```python
from build123d import *

# Parameters (mm, degrees)
F1_DEPTH = 25


with BuildPart() as f1:
    # F0 (on Front) → F1 (new body)
    with BuildSketch(Plane.XZ):
        with BuildLine():
            Line((-24.272264, 6.957319), (-24.272264, -8.5))
            Line((-24.272264, -8.5), (-4.272264, -8.5))
            Line((-4.272264, -8.5), (-4.272264, -5))
            Line((-4.272264, -5), (10.727736, -5))
            Line((10.727736, -5), (10.727736, -11))
            Line((10.727736, -11), (15.727736, -11))
            Line((15.727736, -11), (15.727736, -19.5))
            Line((15.727736, -19.5), (25.727736, -19.5))
            Line((25.727736, -19.5), (25.727736, 19))
            Line((25.727736, 19), (15.727736, 19))
            Line((15.727736, 19), (15.727736, 10))
            Line((15.727736, 10), (10.727736, 10))
            ThreePointArc((10.727736, 10), (9.263269, 6.464466), (5.727736, 5))
            Line((5.727736, 5), (-4.272264, 5))
            Line((-4.272264, 5), (-4.272264, 8.5))
            Line((-4.272264, 8.5), (-20.272264, 8.5))
            Line((-20.272264, 8.5), (-24.272264, 6.957319))
        make_face()
    extrude(amount=F1_DEPTH)


solid = f1.part
```
Work out the finished part from the listing and answer in its coordinate system (mm). A direction names the side the tool comes from. Coordinates: 2 decimals unless noted, no trailing zeros. Write each loop counter-clockwise with the first axis right and the second up, starting at its lowest first coordinate (ties: lowest second). Pieces come first, ordered by that corner, then holes.
Q1. Find the intervals of material crossed by line 1 (X direction, y = -11.75, z = -7); line 2 (X direction, y = -20.25, z = -16); line 3 (Z direction, x = 0, y = -5.5), in increasing order.
Q2. A cutting plane is placed at B-B, the plane z = -9.5. Give the vertices of the cut face in (x, y).
Q3. Which of the six approach directions +Z, -Z, +X, -X, +Y, -Y give full straight-line access (tool end or side, diameter ignored) to faces 1 (the face through (3, -12, -5)), 2 (the face through (15.728, -12, -15)), 3 (the face through (9.3, -12.3, 6.5))?
Q4. Each of these flat-tipped pins is pushed along its axis until it touches: pin 1 Ø6 at (y, z) = (-3, -10) entering from -X; pin 2 Ø5.5 at (x, y) = (12.5, -17) entering from -Z; pin 3 Ø2.5 at (x, y) = (13.5, -6.5) entering from +Z; pin 4 Ø8 at (x, y) = (-1.5, -22.5) entering from -Z. Where does it stop, or does it pass through?
Q5. A cutting plane is placed at A-A, the plane y = -2. Give the vertices of the cut face in (x, z), then the cut area to 3 significant figures.
Q6. A cutting plane is placed at C-C, the plane x = 5. Give the vertices of the cut face in (y, z), then the cut area to 3 significant figures.
Q7. Determine the mould class of faces 4 (the face through (-4.272, -12, 7)), 5 (the face through (10.728, -12, -8)), 6 (the face through (15.728, -12, 15)), 7 (the face through (13, -12, -11)) for opening direction X: released by +X, released by -X, zero draft, split by the parting line, or undercut.
Findings below:
1. line 1: x = -24.27 to -4.27, 10.73 to 25.73
1. line 2: x = 15.73 to 25.73
1. line 3: z = -5 to 5
2. outline: (10.73, -25) - (25.73, -25) - (25.73, 0) - (10.73, 0) - close
3. face 1: -Z, +Y, -Y
3. face 2: -Z, -X, +Y, -Y
3. face 3: +Z, +Y, -Y
4. pin 1: stops at x = -24.27
4. pin 2: stops at z = -11
4. pin 3: stops at z = 10
4. pin 4: stops at z = -8.5
5. outline: (-24.27, -8.5) - (-4.27, -8.5) - (-4.27, -5) - (10.73, -5) - (10.73, -11) - (15.73, -11) - (15.73, -19.5) - (25.73, -19.5) - (25.73, 19) - (15.73, 19) - (15.73, 10) - (10.73, 10) arc R5 cw to (5.73, 5) - (-4.27, 5) - (-4.27, 8.5) - (-20.27, 8.5) - (-24.27, 6.96) - close
5. area: 982 mm2
6. outline: (-25, -5) - (0, -5) - (0, 5) - (-25, 5) - close
6. area: 250 mm2
7. face 4: undercut
7. face 5: undercut
7. face 6: released by -X
7. face 7: zero draft
